Part model, mm, in its own coordinate system. Face numbers are marked on the shaded views. Coordinates: 2 decimals unless noted, no trailing zeros. Loops run counter-clockwise (first coordinate to the right, second up) from the corner with the lowest first, then second, coordinate; pieces in that order, holes last. Notation, with made-up numbers: M 2,59.5 L 28,59.5 A17 cw 28,64.5 Z; hole C 81,-40 d6. An arc over 180 degrees is marked long. Use a Markdown table: item, result. Add a question column.
1) Pull direction Y, two halves, no side cores. Call the marked faces 1, 2 and 3: released by +Y, released by -Y, zero draft, split by the parting line, or undercut.
2) Band-saw the part on A-A (z = 14). List the corners of the cut face in (x, y), plus the area to 3 significant figures.
3) Wall check: probe 1 along X at (y, z) = (-0.5, 11.5); probe 2 along Y at (x, z) = (0, 29); probe 3 along X at (y, z) = (-29, 1). Give the ranges that are in metal, low to high. Write a range as from..to.
4) Band-saw the part on C-C (y = -26). State how many separate pieces and enclosed holes the cut face has, plus the area to 3 significant figures.
5) Pin check, flat tips, straight feed: pin 1 Ø1 at (y, z) = (-5.5, 23) entering from -X; pin 2 Ø6 at (x, z) = (-4.5, 32.5) entering from -Y; pin 3 Ø6 at (x, z) = (-9.5, 30) entering from -Y; pin 4 Ø8.5 at (x, y) = (-9.525, -29.21) entering from +Z. Stop position of each tip, or through.
6) Band-saw the part on B-B (y = 0). List the corners of the cut face in (x, z) (3 decimals), plus the area to 3 significant figures.
from build123d import *

# Parameters (mm, degrees)
F0_R     = 39.497
F1_DEPTH = 38.1
F2_R     = 36.957
F3_DEPTH = 35.56
F4_R     = 0.762
F5_R     = 0.762
F7_DEPTH = 25.4
F9_DEPTH = 25.4


with BuildPart() as f1:
    # F0 (on Top) → F1 (new body)
    with BuildSketch(Plane.XY):
        Circle(F0_R)
    extrude(amount=F1_DEPTH)

    # F2 (on face) → F3 (cut)
    with BuildSketch(Plane.XY.offset(38.1)):
        Circle(F2_R)
    extrude(amount=-F3_DEPTH, mode=Mode.SUBTRACT)

    # F4
    f4_edges = [f1.edges().sort_by_distance(p)[0] for p in [
        (-36.957, 0, 2.54),
    ]]
    fillet(f4_edges, radius=F4_R)

    # F5
    f5_edges = [f1.edges().sort_by_distance(p)[0] for p in [
        (-39.497, 0, 38.1),
    ]]
    fillet(f5_edges, radius=F5_R)

    # F6 (on face) → F7 (cut)
    with BuildSketch(Plane(origin=(0, 0, 0), x_dir=(1, 0, 0), z_dir=(0, 0, -1))):
        with BuildLine():
            Line((0, -25.019), (0, -30.353))
            Line((0, -30.353), (0, -35.687))
            ThreePointArc((0, -35.687), (3.771708, -34.124708), (5.334, -30.353))
            ThreePointArc((5.334, -30.353), (3.771708, -26.581292), (0, -25.019))
        make_face()
        with BuildLine():
            Line((0, -35.687), (0, -30.353))
            Line((0, -30.353), (0, -25.019))
            ThreePointArc((0, -25.019), (-5.334, -30.353), (0, -35.687))
        make_face()
    extrude(amount=-F7_DEPTH, mode=Mode.SUBTRACT)

    # F8 (on face) → F9 (cut)
    with BuildSketch(Plane(origin=(0, 0, 0), x_dir=(1, 0, 0), z_dir=(0, 0, -1))):
        with BuildLine():
            ThreePointArc((14.859, 29.21), (9.525, 34.544), (4.191, 29.21))
            ThreePointArc((4.191, 29.21), (9.525, 23.876), (14.859, 29.21))
        make_face()
        with BuildLine():
            ThreePointArc((-4.191, 29.21), (-13.841951, 32.342969), (-7.87135, 24.138807))
            Line((-7.87135, 24.138807), (-9.525, 29.21))
            Line((-9.525, 29.21), (-4.191, 29.21))
        make_face()
        with BuildLine():
            Line((-9.525, 29.21), (-7.87135, 24.138807))
            ThreePointArc((-7.87135, 24.138807), (-5.208049, 26.077031), (-4.191, 29.21))
            Line((-4.191, 29.21), (-9.525, 29.21))
        make_face()
    extrude(amount=-F9_DEPTH, mode=Mode.SUBTRACT)


solid = f1.part
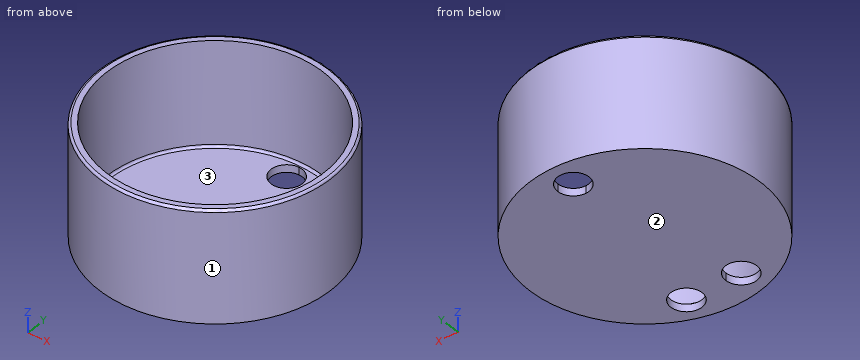
Entries:
| question | item | result |
|---|---|---|
| 1 | face 1 | split by the parting line |
| 1 | face 2 | zero draft |
| 1 | face 3 | undercut |
| 2 | outline | C 0,0 d78.99; hole C 0,0 d73.91 |
| 2 | area | 610 mm2 |
| 3 | probe 1 | -39.49..-36.95, 36.95..39.49 |
| 3 | probe 2 | -39.5..-36.96, 36.96..39.5 |
| 3 | probe 3 | -26.81..-14.85, -4.2..4.2, 14.85..26.81 |
| 4 | separate pieces | 3 |
| 4 | enclosed holes | 0 |
| 4 | area | 354 mm2 |
| 5 | pin 1 | x = -39.18 |
| 5 | pin 2 | y = -39.47 |
| 5 | pin 3 | y = -38.96 |
| 5 | pin 4 | through |
| 6 | outline | M -39.497,0 L 39.497,0 L 39.497,37.338 A0.762 ccw 38.735,38.1 L 36.957,38.1 L 36.957,3.302 A0.762 cw 36.195,2.54 L -36.195,2.54 A0.762 cw -36.957,3.302 L -36.957,38.1 L -38.735,38.1 A0.762 ccw -39.497,37.338 Z |
| 6 | area | 381 mm2 |
